Geometry: see drawing. Coordinates: mm, zero at the bounding-box minimum. A direction names the side the tool comes from. Coordinates: 2 decimals unless noted, no trailing zeros. Write each loop counter-clockwise with the first axis right and the second up, starting at its lowest first coordinate (ties: lowest second). Pieces come first, ordered by that corner, then holes. Notation, with made-up numbers: (70.25, -28.75) -> (77.25, -28.75) arc R10 cw to (77.25, -24.75) -> close; hole circle Ø7 at (19, 54). An arc over 180 degrees is marked (long way). Use one line per item in the form item = value. Start each with the question number.
(1) Set-up query: the marked faces 1, 2 and 3. Return all of +Z, -Z, +X, -X, +Y, -Y with unobstructed straight access to the full face (end or side cutting, diameter ignored); none if empty.
(2) Cut plane D-D on x = 8. Return the cut outline in (y, z), plus the area to 4 significant figures.
(3) Ray query, line 1 along Z through (x, y) = (51, 10.5); line 2 along Y through (x, z) = (62.5, 6.5). Return the intervals inside material, ascending.
(4) Cut plane B-B on x = 62. Return the cut outline in (y, z).
(5) First-contact query: pin 1 (8 mm diameter, centred on x = 41, y = 16.5, fed in from -Z); pin 2 (10 mm diameter, centred on x = 49.5, y = 15.5, fed in from +Z). Flat tips, straight axial feed; report the tip coordinate or a pass-through.
(6) Cut plane A-A on y = 11.25. Return the cut outline in (x, z) (1 decimal).
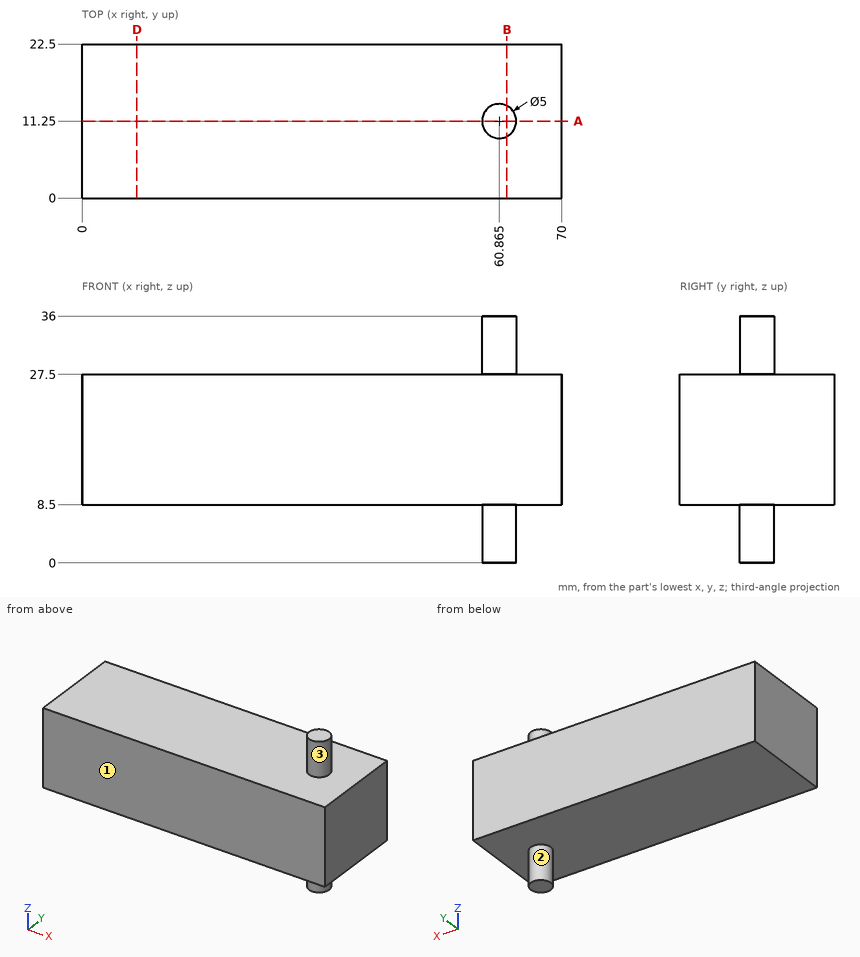
Values:
q1.face_1 = +Z, -Z, +X, -X, -Y
q1.face_2 = -Z
q1.face_3 = +Z
q2.outline = (0, 8.5) -> (22.5, 8.5) -> (22.5, 27.5) -> (0, 27.5) -> close
q2.area = 427.5 mm2
q3.line_1 = 8.5 to 27.5
q3.line_2 = 9.36 to 13.14
q4.outline = (0, 8.5) -> (9.02, 8.5) -> (9.02, 0) -> (13.48, 0) -> (13.48, 8.5) -> (22.5, 8.5) -> (22.5, 27.5) -> (13.48, 27.5) -> (13.48, 36) -> (9.02, 36) -> (9.02, 27.5) -> (0, 27.5) -> close
q5.pin_1 = 8.5
q5.pin_2 = 27.5
q6.outline = (0, 8.5) -> (58.4, 8.5) -> (58.4, 0) -> (63.4, 0) -> (63.4, 8.5) -> (70, 8.5) -> (70, 27.5) -> (63.4, 27.5) -> (63.4, 36) -> (58.4, 36) -> (58.4, 27.5) -> (0, 27.5) -> close
